from build123d import *

# Parameters (mm, degrees)
SKETCH1_W           = 7.62
SKETCH1_H           = 19.05
BOSS_EXTRUDE1_DEPTH = 63.5
SKETCH2_R           = 0.889
CUT_EXTRUDE1_DEPTH  = 6.35
SKETCH3_R           = 3.3782
CUT_EXTRUDE2_DEPTH  = 8.62
SKETCH4_R           = 3.3782
CUT_EXTRUDE3_DEPTH  = 8.62
SKETCH5_R           = 5.334
CUT_EXTRUDE4_DEPTH  = 8.62


with BuildPart() as part:
    # Sketch1 → Boss-Extrude1 (new body)
    with BuildSketch(Plane.XY):
        with Locations((3.81, 9.525)):
            Rectangle(SKETCH1_W, SKETCH1_H)
    extrude(amount=-BOSS_EXTRUDE1_DEPTH)

    # Sketch2 → Cut-Extrude1 (cut)
    with BuildSketch(Plane.XY):
        with Locations((2.032, 11.43)):
            Circle(SKETCH2_R)
    extrude(amount=-CUT_EXTRUDE1_DEPTH, mode=Mode.SUBTRACT)

    # Sketch3 → Cut-Extrude2 (cut, through all)
    with BuildSketch(Plane.ZY):
        with Locations((-48.26, 12.7)):
            Circle(SKETCH3_R)
    extrude(amount=-CUT_EXTRUDE2_DEPTH, mode=Mode.SUBTRACT)

    # Sketch4 → Cut-Extrude3 (cut, through all)
    with BuildSketch(Plane.ZY):
        with Locations((-26.67, 12.7)):
            Circle(SKETCH4_R)
    extrude(amount=-CUT_EXTRUDE3_DEPTH, mode=Mode.SUBTRACT)

    # Sketch5 → Cut-Extrude4 (cut, through all)
    with BuildSketch(Plane.ZY):
        with Locations((-11.049, 11.43)):
            Circle(SKETCH5_R)
    extrude(amount=-CUT_EXTRUDE4_DEPTH, mode=Mode.SUBTRACT)


solid = part.part
Model file for the job. Use its own axes, mm. A direction names the side the tool comes from. Give positions to 0.01 mm unless a question says otherwise; leave off trailing zeros. Write each loop counter-clockwise with the first axis right and the second up, starting at its lowest first coordinate (ties: lowest second). Pieces come first, ordered by that corner, then holes. Notation, with made-up numbers: M -3,8 L 9,8 A13 cw 9,25 Z; hole C -36,-18.5 d2. An arc over 180 degrees is marked long. One line per item, written item: value. Start each with the question number.
Q1. 3-axis set-ups, long thin cutter, end or side, ignore diameter. For faces 4 (the flat face through (4, 0, -31)), 5 (the cylindrical face through (2.853, 11.09, -2.854)): which of +Z, -Z, +X, -X, +Y, -Y reach the whole face in a straight line?
Q2. Drop flat-ended pins along their axis: pin 1 Ø1.1 at (x, y) = (2.032, 11.43) entering from +Z; pin 2 Ø2 at (y, z) = (10.5, -7) entering from -X. Give the stop position or say it passes through.
Q3. Saw through at C-C, the plane x = 2.25. Write the cut outline in (y, z).
Q4. Probe probe 1 along Z at (x, y) = (1, 13.75); probe 2 along Y at (x, z) = (2.5, -48.26); probe 3 along Z at (x, y) = (1, 11.25). List the from-to ranges inside material, lowest first. Write a range as [from, to].
Q5. Saw through at A-A, the plane z = -26.67. Write the cut outline in (x, y).
Q6. Two-plate mould, pull along Y, no slides. Class faces 1 (the flat face through (0, 9, -31)), 2 (the cylindrical face through (3.757, 13.715, -45.038)), 3 (the flat face through (4, 19.05, -31)): +Y half, -Y half, draft (parallel to the pull), parting line (faces both ways), or undercut.
Q7. Saw through at B-B, the plane y = 13.75. Write the cut outline in (x, z).
Output values:
1. face 4: +Z, -Z, +X, -X, -Y
1. face 5: +Z
2. pin 1: stops at z = -16.35
2. pin 2: passes through
3. outline: M 0,-63.5 L 19.05,-63.5 L 19.05,0 L 12.29,0 L 12.29,-5.79 A5.33 cw long 10.57,-5.79 L 10.57,0 L 0,0 Z; hole C 12.7,-48.26 d6.76; hole C 12.7,-26.67 d6.76
4. probe 1: z = [-63.5, -51.47], [-45.05, -29.88], [-23.46, -15.85], [-6.25, 0]
4. probe 2: y = [0, 9.32], [16.08, 19.05]
4. probe 3: z = [-63.5, -51.31], [-45.21, -29.72], [-23.62, -16.38], [-5.72, 0]
5. outline: M 0,0 L 7.62,0 L 7.62,9.32 L 0,9.32 Z; M 0,16.08 L 7.62,16.08 L 7.62,19.05 L 0,19.05 Z
6. face 1: draft
6. face 2: undercut
6. face 3: +Y half
7. outline: M 0,-63.5 L 7.62,-63.5 L 7.62,-51.47 L 0,-51.47 Z; M 0,-45.05 L 7.62,-45.05 L 7.62,-29.88 L 0,-29.88 Z; M 0,-23.46 L 7.62,-23.46 L 7.62,-15.85 L 0,-15.85 Z; M 0,-6.25 L 7.62,-6.25 L 7.62,0 L 0,0 Z
